```python
from build123d import *

# Parameters (mm, degrees)
SKETCH_1_W          = 15
SKETCH_1_H          = 135
SKETCH_1_W_2        = 40
SKETCH_1_H_2        = 10
EXTRUDE_1_DEPTH     = 12
SKETCH_2_R          = 4
EXTRUDE_2_DEPTH     = 185
SKETCH_3_R          = 1.75
CUT_EXTRUDE_1_DEPTH = 235.166607355
FILLET_1_R          = 3
FILLET_2_R          = 5
FILLET_3_R          = 1


with BuildPart() as part:
    # ｽｹｯﾁ1 → ﾎﾞｽ - 押し出し1 (new body)
    with BuildSketch(Plane.XY):
        Rectangle(SKETCH_1_W, SKETCH_1_H)
        with Locations((0, -62.5)):
            Rectangle(SKETCH_1_W_2, SKETCH_1_H_2)
    extrude(amount=EXTRUDE_1_DEPTH)

    # ｽｹｯﾁ2 → ﾎﾞｽ - 押し出し2 (add)
    with BuildSketch(Plane.XY.offset(12)):
        with Locations(Location((0, 12.5, 0), (0, 0, 180))):
            Circle(SKETCH_2_R)
        with Locations(Location((0, 62.5, 0), (0, 0, 180))):
            Circle(SKETCH_2_R)
    extrude(amount=EXTRUDE_2_DEPTH)

    # ｽｹｯﾁ3 → ｶｯﾄ - 押し出し1 (cut, through all)
    with BuildSketch(Plane(origin=(0, -57.5, 0), x_dir=(1, 0, 0), z_dir=(0, 1, 0))):
        with Locations(Location((-15, -6, 0), (0, 0, 270))):
            Circle(SKETCH_3_R)
        with Locations(Location((15, -6, 0), (0, 0, 270))):
            Circle(SKETCH_3_R)
    extrude(amount=-CUT_EXTRUDE_1_DEPTH, mode=Mode.SUBTRACT)

    # ﾌｨﾚｯﾄ1
    fillet_1_edges = [part.edges().sort_by_distance(p)[0] for p in [
        (-7.5, -57.5, 6),
        (7.5, -57.5, 6),
    ]]
    fillet(fillet_1_edges, radius=FILLET_1_R)

    # ﾌｨﾚｯﾄ2
    fillet_2_edges = [part.edges().sort_by_distance(p)[0] for p in [
        (7.5, 67.5, 6),
        (-7.5, 67.5, 6),
    ]]
    fillet(fillet_2_edges, radius=FILLET_2_R)

    # ﾌｨﾚｯﾄ3
    fillet_3_edges = [part.edges().sort_by_distance(p)[0] for p in [
        (20, -57.5, 6),
        (-20, -57.5, 6),
        (-15.25, -57.5, 12),
        (20, -62.5, 12),
        (-20, -62.5, 12),
        (-15.25, -57.5, 0),
        (20, -62.5, 0),
        (-20, -62.5, 0),
        (7.5, 4, 12),
        (7.5, 4, 0),
        (15.25, -57.5, 12),
        (15.25, -57.5, 0),
        (-7.5, 4, 12),
        (-7.5, 4, 0),
        (8.378679656, -56.621320344, 0),
        (8.378679656, -56.621320344, 12),
        (-8.378679656, -56.621320344, 0),
        (-8.378679656, -56.621320344, 12),
        (0, 67.5, 0),
        (0, 67.5, 12),
        (-6.035533906, 66.035533906, 0),
        (6.035533906, 66.035533906, 0),
        (-6.035533906, 66.035533906, 12),
        (6.035533906, 66.035533906, 12),
    ]]
    fillet(fillet_3_edges, radius=FILLET_3_R - 0.0001)  # a hair under: the kernel refuses the full size


solid = part.part
```
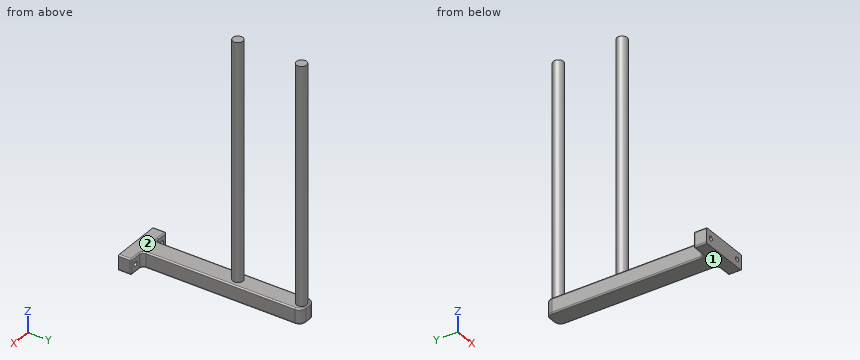
CAD build for the part. Positions are in the model's coordinates, mm. Face numbers are marked on the shaded views. Round coordinates to 2 decimals unless told otherwise and drop trailing zeros. Write each loop counter-clockwise with the first axis right and the second up, starting at its lowest first coordinate (ties: lowest second). Pieces come first, ordered by that corner, then holes.
Item 1: Band-saw the part on D-D on y = -45.5. Write the cut outline in (x, z).
Filled in:
outline: (-7.5, 1) arc R1 ccw to (-6.5, 0) - (6.5, 0) arc R1 ccw to (7.5, 1) - (7.5, 11) arc R1 ccw to (6.5, 12) - (-6.5, 12) arc R1 ccw to (-7.5, 11) - close
Item 2: Band-saw the part on C-C on z = 64. Write the cut outline in (x, y), then the cut area to 3 significant figures.
Filled in:
outline: circle Ø8 at (0, 12.5); circle Ø8 at (0, 62.5)
area: 101 mm2
Item 3: Band-saw the part on B-B on y = 12.5. Write the cut outline in (x, z).
Filled in:
outline: (-7.5, 1) arc R1 ccw to (-6.5, 0) - (6.5, 0) arc R1 ccw to (7.5, 1) - (7.5, 11) arc R1 ccw to (6.5, 12) - (4, 12) - (4, 197) - (-4, 197) - (-4, 12) - (-6.5, 12) arc R1 ccw to (-7.5, 11) - close
Item 4: Drop flat-ended pins along their axis: pin 1 Ø5 at (y, z) = (16.5, 6) entering from +X; pin 2 Ø5.5 at (x, z) = (15, 6) entering from +Y; pin 3 Ø8 at (y, z) = (3.5, 8) entering from -X. Give the stop position or say it passes through.
Filled in:
pin 1: stops at x = 7.5
pin 2: stops at y = -57.5
pin 3: stops at x = -7.5
Item 5: Drill centre lines: L1, parallel to X at y = -60, z = 6; L2, parallel to Y at x = 0.5, z = 120; L3, parallel to Z at x = 17.5, y = -60. Where is each one in solid material? Low to high.
Filled in:
L1: x = -20 to -16.75, -13.25 to 13.25, 16.75 to 20
L2: y = 8.53 to 16.47, 58.53 to 66.47
L3: z = 0 to 12
Item 6: Mould opens along Y. For the marked faces 1 and 2 say: released by +Y, released by -Y, zero draft, split by the parting line, or undercut.
Filled in:
face 1: zero draft
face 2: undercut
